CAD build for the part. Positions are in the model's coordinates, mm. Round coordinates to 2 decimals unless told otherwise and drop trailing zeros. Write each loop counter-clockwise with the first axis right and the second up, starting at its lowest first coordinate (ties: lowest second). Pieces come first, ordered by that corner, then holes. Notation, with made-up numbers: (33, 86) - (53, 86) arc R17 ccw to (53, 98) - close; hole circle Ø9 at (58.25, 25). An arc over 180 degrees is marked (long way). Answer in a Markdown table with one row per item.
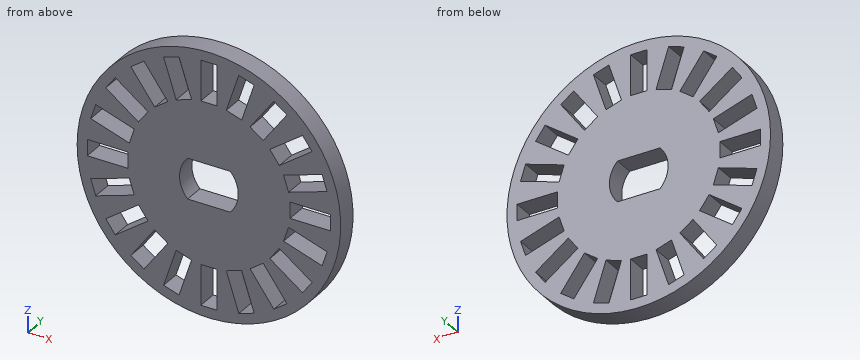
Autodesk Inventor part; units mm, degrees
ref_plane "YZ Plane" through (0, 0, 0) normal (1, 0, 0) x (0, 1, 0)
ref_plane "XZ Plane" through (0, 0, 0) normal (0, 1, 0) x (-1, 0, 0)
ref_plane "XY Plane" through (0, 0, 0) normal (0, 0, 1) x (1, 0, 0)
sketch "Esboço1" plane through (0, 0, 0) normal (0, 1, 0) x (-1, 0, 0)
  line L0 (-2.1, 2) -> (2.1, 2)
  line L1 (-2.1, -2) -> (2.1, -2)
  arc A0 (-2.1, 2) -> (-2.1, -2) centre (0, 0) ccw
  arc A1 (2.1, -2) -> (2.1, 2) centre (0, 0) ccw
  circle A2 centre (0, 0) radius 13
  line L2 (0, -18.2) -> (0, 18.2)
  dimension "d2" = 2
  dimension "d3" = 2
  dimension "d4" = 2.9
  dimension "d5" = 2.9
  dimension "d40" = 2
  dimension "d41" = 26
extrude "Extrusão4" add sketch "Esboço1" along normal blind 2 contours A0 L1 L2 A2 L0 | L2 A2 L1 A1 L0
sketch "Esboço17" plane through (0, 0, 0) normal (0, -1, 0) x (1, 0, 0)
  line L0 (-0.8, 12) -> (0.8, 12)
  line L1 (0.8, 12) -> (0.8, 8)
  line L2 (0.8, 8) -> (-0.8, 8)
  line L3 (-0.8, 8) -> (-0.8, 12)
  line L4 (0, 18.2) -> (0, -18.2)
  point P0 (0, 0)
  point P1 (0, 8)
  dimension "d114" = 8
  dimension "d115" = 4
  dimension "d116" = 0.8
  dimension "d117" = 0.8
extrude "Extrusão14" cut sketch "Esboço17" against normal through all
pattern_circular "Padrão circular10" count 20 over 360 about axis through (0, 0, 0) along (0, 1, 0) of "Extrusão14"
ref_plane "Plano de trabalho4" through (0, 1, 0) normal (0, -1, 0) x (1, 0, 0)
equation "\"d2\" = d40"
equation "\"d4\" = d5"
equation "\"d117\" = d116"
properties part number "Encoder Disco-Novo-12-furos-04"
Q1. Saw through at B-B on x = 0. List the corners of the cut face in (y, z), then the cut area to 3 significant figures.
Computed:
| item | result |
|---|---|
| outline | (0, -13) - (2, -13) - (2, -12) - (0, -12) - close; (0, -8) - (2, -8) - (2, -2) - (0, -2) - close; (0, 2) - (2, 2) - (2, 8) - (0, 8) - close; (0, 12) - (2, 12) - (2, 13) - (0, 13) - close |
| area | 28.0 mm2 |
Q2. Drill centre lines: line 1 (X direction, y = 1.95, z = -0.75); line 2 (X direction, y = 1.1, z = -9); line 3 (Z direction, x = -8.75, y = 1.1). Where is each one in solid material? Low to high.
Computed:
| item | result |
|---|---|
| line 1 | x = -12.98 to -12, -8 to -2.8, 2.8 to 8, 12 to 12.98 |
| line 2 | x = -9.38 to -7.53, -5.55 to -3.77, -2.08 to -0.8, 0.8 to 2.08, 3.77 to 5.55, 7.53 to 9.38 |
| line 3 | z = -9.61 to -7.35, -5.37 to -3.68, -2 to -0.8, 0.8 to 2, 3.68 to 5.37, 7.35 to 9.61 |
Q3. Saw through at C-C on y = 0.7. Count the separate pieces of the cut face and the enclosed holes in it, then the cut area to 3 significant figures.
Computed:
| item | result |
|---|---|
| separate pieces | 1 |
| enclosed holes | 21 |
| area | 382 mm2 |
Q4. Flat gauge pins, fed straight in: pin 1 (1 mm diameter, centred on y = 1.5, z = -9.5, fed in from +X); pin 2 (0.5 mm diameter, centred on y = 0.5, z = -0.5, fed in from +X); pin 3 (0.5 mm diameter, centred on x = -0.5, y = 1, fed in from -Z). Where does each tip first touch, or does it go through?
Computed:
| item | result |
|---|---|
| pin 1 | stops at x = 9.38 |
| pin 2 | stops at x = 13 |
| pin 3 | stops at z = -13 |
Q5. Saw through at A-A on z = 0. List the corners of the cut face in (x, y), then the cut area to 3 significant figures.
Computed:
| item | result |
|---|---|
| outline | (-13, 0) - (-12, 0) - (-12, 2) - (-13, 2) - close; (-8, 0) - (-2.9, 0) - (-2.9, 2) - (-8, 2) - close; (2.9, 0) - (8, 0) - (8, 2) - (2.9, 2) - close; (12, 0) - (13, 0) - (13, 2) - (12, 2) - close |
| area | 24.4 mm2 |
